CAD build for the part. Positions are in the model's coordinates, mm. Coordinates: 2 decimals unless noted, no trailing zeros. Loops run counter-clockwise (first coordinate to the right, second up) from the corner with the lowest first, then second, coordinate; pieces in that order, holes last. Notation, with made-up numbers: (-19.5, 2) -> (31.5, 2) arc R12 ccw to (31.5, 21) -> close; hole circle Ø5 at (60.5, 12.5). An arc over 180 degrees is marked (long way). Return JSON: item names as keys, results as strings. Group by question number.
(1) Saw through at D-D on y = 1.9. Give the number of separate pieces and of enclosed holes in the cut face, then the cut area to 3 significant figures.
(2) Saw through at C-C on z = -6.5. Write the cut outline in (x, y).
(3) Probe L1, parallel to X at y = 2.3, z = -11; L2, parallel to Z at x = -1.75, y = 1; L3, parallel to Z at x = -0.25, y = 1.6. List the from-to ranges inside material, lowest first.
(4) Saw through at A-A on z = 40.5. Write the cut outline in (x, y).
(5) Saw through at B-B on z = 22.5. Write the cut outline in (x, y), then the cut area to 3 significant figures.
(6) Flat gauge pins, fed straight in: pin 1 Ø1.8 at (x, z) = (0, 33.5) entering from +Y; pin 2 Ø1.5 at (y, z) = (2, 67.5) entering from -X; pin 3 Ø1.5 at (y, z) = (1, 66) entering from +X. Where does each tip first touch, or does it go through?
```python
from build123d import *

# Parameters (mm, degrees)
SKETCH_1_W          = 25.2
SKETCH_1_H          = 28
EXTRUDE_1_DEPTH     = 3
SKETCH_4_R          = 1.5
SKETCH_4_W          = 16
SKETCH_4_H          = 16
CUT_EXTRUDE_3_DEPTH = 20.072493282
SKETCH_6_W          = 30
SKETCH_6_H          = 37.5
EXTRUDE_2_DEPTH     = 3
SKETCH_7_R          = 1.5
CUT_EXTRUDE_5_DEPTH = 54.723830839
FILLET_1_R          = 10
SKETCH_8_W          = 17
SKETCH_8_H          = 16
CUT_EXTRUDE_6_DEPTH = 54.723830839
FILLET_2_R          = 3
SKETCH_5_R          = 1.5
SKETCH_5_R_2        = 1.275
CUT_EXTRUDE_7_DEPTH = 10
SKETCH_9_W          = 20
SKETCH_9_H          = 3
EXTRUDE_3_DEPTH     = 25
FILLET_3_R          = 12
SKETCH_12_R         = 1.5
CUT_EXTRUDE_9_DEPTH = 79.014421744


with BuildPart() as part:
    # 草图1 → 凸台-拉伸1 (new body)
    with BuildSketch(Plane(origin=(0, 0, 0), x_dir=(1, 0, 0), z_dir=(0, 1, 0))):
        Rectangle(SKETCH_1_W, SKETCH_1_H)
    extrude(amount=EXTRUDE_1_DEPTH)

    # 草图4 → 切除-拉伸3 (cut, through all)
    with BuildSketch(Plane(origin=(0, 3, 0), x_dir=(1, 0, 0), z_dir=(0, 1, 0))):
        with Locations(Location((4, 11, 0), (0, 0, 270))):
            Circle(SKETCH_4_R)
        with Locations(Location((-4, 11, 0), (0, 0, 270))):
            Circle(SKETCH_4_R)
        Rectangle(SKETCH_4_W, SKETCH_4_H)
    extrude(amount=-CUT_EXTRUDE_3_DEPTH, mode=Mode.SUBTRACT)

    # 草图6 → 凸台-拉伸2 (add)
    with BuildSketch(Plane(origin=(0, 3, 0), x_dir=(1, 0, 0), z_dir=(0, 1, 0))):
        with Locations((0, -32.75)):
            Rectangle(SKETCH_6_W, SKETCH_6_H)
    extrude(amount=-EXTRUDE_2_DEPTH)

    # 草图7 → 切除-拉伸5 (cut, through all)
    with BuildSketch(Plane(origin=(0, 3, 0), x_dir=(1, 0, 0), z_dir=(0, 1, 0))):
        with Locations(Location((0, -33.5, 0), (0, 0, 270))):
            Circle(SKETCH_7_R)
        with Locations(Location((-5, -40.5, 0), (0, 0, 270))):
            Circle(SKETCH_7_R)
        with Locations(Location((5, -40.5, 0), (0, 0, 270))):
            Circle(SKETCH_7_R)
        with Locations(Location((0, -47.5, 0), (0, 0, 270))):
            Circle(SKETCH_7_R)
    extrude(amount=-CUT_EXTRUDE_5_DEPTH, mode=Mode.SUBTRACT)

    # 圆角1
    # the kernel refuses this fillet: 10 mm, written as the material it adds along each edge
    with BuildSketch(Plane(origin=(12.6, 0, 14), x_dir=(0, 0, -1), z_dir=(0, 1, 0))) as fillet_1_piece_1:
        with BuildLine():
            CenterArc((6.499230724, -10), FILLET_1_R, 90, 40.535802111)
            Line((0, -2.4), (-0.129984614, -2.248))
            ThreePointArc((-0.129984614, -2.248), (-0.2, -1.2), (-0.2, 0))
            Line((-0.2, 0), (0, 0.2))
            Line((0, 0.2), (6.499230724, 0.2))
            Line((6.499230724, 0.2), (6.499230724, 0))
        make_face()
    extrude(amount=3)
    with BuildSketch(Plane(origin=(-12.6, 0, 14), x_dir=(-1, 0, 0), z_dir=(0, 1, 0))) as fillet_1_piece_2:
        with BuildLine():
            CenterArc((10, -6.499230724), FILLET_1_R, 139.464197889, 40.535802111)
            Line((0, -6.499230724), (-0.2, -6.499230724))
            Line((-0.2, -6.499230724), (-0.2, 0))
            Line((-0.2, 0), (0, 0.2))
            ThreePointArc((0, 0.2), (1.2, 0.2), (2.248, 0.129984614))
            Line((2.248, 0.129984614), (2.4, 0))
        make_face()
    extrude(amount=3)

    # 草图8 → 切除-拉伸6 (cut, through all)
    with BuildSketch(Plane(origin=(0, 3, 0), x_dir=(1, 0, 0), z_dir=(0, 1, 0))):
        with Locations((0, -20)):
            Rectangle(SKETCH_8_W, SKETCH_8_H)
    extrude(amount=-CUT_EXTRUDE_6_DEPTH, mode=Mode.SUBTRACT)

    # 圆角2
    fillet_2_edges = [part.edges().sort_by_distance(p)[0] for p in [
        (8.5, 1.5, 12),
        (8.5, 1.5, 28),
        (-8.5, 1.5, 28),
        (-8.5, 1.5, 12),
    ]]
    fillet(fillet_2_edges, radius=FILLET_2_R)

    # 草图5 → 切除-拉伸7 (cut)
    with BuildSketch(Plane(origin=(0, 3, 0), x_dir=(1, 0, 0), z_dir=(0, 1, 0))):
        with Locations((8, 6.5)):
            Circle(SKETCH_5_R)
        with Locations((-8, 6.5)):
            Circle(SKETCH_5_R)
        with Locations((8, -6.5)):
            Circle(SKETCH_5_R)
        with Locations((-8, -6.725)):
            Circle(SKETCH_5_R_2)
    extrude(amount=-CUT_EXTRUDE_7_DEPTH, mode=Mode.SUBTRACT)

    # 草图9 → 凸台-拉伸3 (add)
    with BuildSketch(Plane.XY.offset(51.5)):
        with Locations((0, 1.5)):
            Rectangle(SKETCH_9_W, SKETCH_9_H)
    extrude(amount=EXTRUDE_3_DEPTH)

    # 圆角3
    # the kernel refuses this fillet: 12 mm, written as the material it adds along each edge
    with BuildSketch(Plane(origin=(10, 3, 51.5), x_dir=(1, 0, 0), z_dir=(0, -1, 0)), Plane(origin=(-10, 0, 51.5), x_dir=(-1, 0, 0), z_dir=(0, 1, 0))) as fillet_3_piece_1:
        with BuildLine():
            CenterArc((12, 9.746794345), FILLET_3_R, 180, 54.314665287)
            Line((0, 9.746794345), (-0.24, 9.746794345))
            Line((-0.24, 9.746794345), (-0.24, 0))
            Line((-0.24, 0), (0, -0.24))
            ThreePointArc((0, -0.24), (2.5, -0.24), (4.86, -0.194935887))
            Line((4.86, -0.194935887), (5, 0))
        make_face()
    extrude(amount=3)

    # 草图12 → 切除-拉伸9 (cut, through all)
    with BuildSketch(Plane(origin=(0, 3, 0), x_dir=(1, 0, 0), z_dir=(0, 1, 0))):
        with Locations(Location((5, -71.5, 0), (0, 0, 270))):
            Circle(SKETCH_12_R)
        with Locations(Location((-5, -71.5, 0), (0, 0, 270))):
            Circle(SKETCH_12_R)
    extrude(amount=-CUT_EXTRUDE_9_DEPTH, mode=Mode.SUBTRACT)


solid = part.part
```
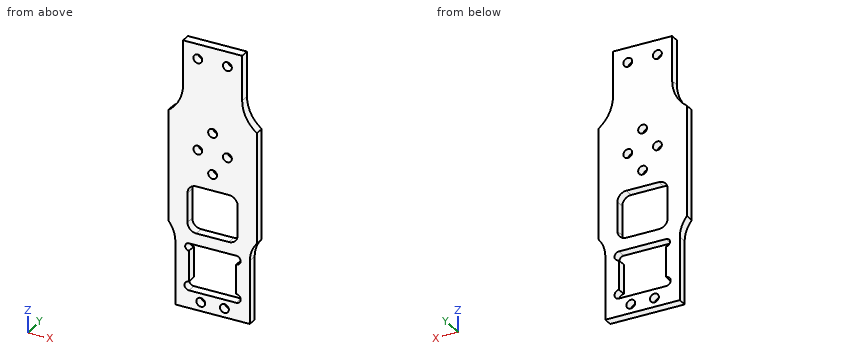
Geometry results:
{
 "1": {"separate pieces": "1", "enclosed holes": "10", "area": "1,780 mm²"},
 "2": {"outline": "(-12.6, 0) -> (-9.5, 0) -> (-9.5, 3) -> (-12.6, 3) -> close; (9.5, 0) -> (12.6, 0) -> (12.6, 3) -> (9.5, 3) -> close"},
 "3": {"L1": "-12.6 to -5.5, -2.5 to 2.5, 5.5 to 12.6", "L2": "-14 to -8, 8 to 12, 28 to 76.5", "L3": "-14 to -8, 8 to 12, 28 to 32.02, 34.98 to 46.02, 48.98 to 76.5"},
 "4": {"outline": "(-15, 0) -> (-6.5, 0) -> (-6.5, 3) -> (-15, 3) -> close; (-3.5, 0) -> (3.5, 0) -> (3.5, 3) -> (-3.5, 3) -> close; (6.5, 0) -> (15, 0) -> (15, 3) -> (6.5, 3) -> close"},
 "5": {"outline": "(-15, 0) -> (-8.5, 0) -> (-8.5, 3) -> (-15, 3) -> close; (8.5, 0) -> (15, 0) -> (15, 3) -> (8.5, 3) -> close", "area": "39.0 mm²"},
 "6": {"pin 1": "through", "pin 2": "x = -10", "pin 3": "x = 10"}
}
